For this review, use the dimensioned drawing (mm, ordinates from the lowest corner) and the shaded views. Coordinates: 2 decimals unless noted, no trailing zeros. Order: outer loops, then holes, each group sorted by start corner. A loop starts at its lowest first (then second) coordinate and runs counter-clockwise, first axis right, second up. Notation, with made-up numbers: M -33,1 L 18,1 A22 ccw 18,35 Z; hole C 76.25,69.5 d1. An arc over 180 degrees is marked long. Answer as CSV lines item,"result". Start each with the question number.
Q1. The part is to be moulded in two halves that separate along Y. For the marked faces 1, 2 and 3, say which applies: +Y half, -Y half, draft (parallel to the pull), parting line (faces both ways), or undercut.
Q2. For P1, Ø4, axis at x = 50.5, z = 34.5, coming from the -Y side; P2, Ø1.5, axis at x = 84, y = 220, coming from the +Z side; P3, Ø3, axis at x = 40, y = 187.5, coming from the +Z side, all flat-tipped, find the tip position at first contact; note any pin that passes through.
Q3. Wall thickness on L1, parallel to Y at x = 26, z = 150; L2, parallel to Y at x = 19.5, z = 120.5; L3, parallel to Z at x = 37, y = 148: over which ranges is each line inside the solid? List them lowest first. Write a range as [from, to].
Q4. Consider section A-A on z = 150. Write out the cut boundary in (x, y).
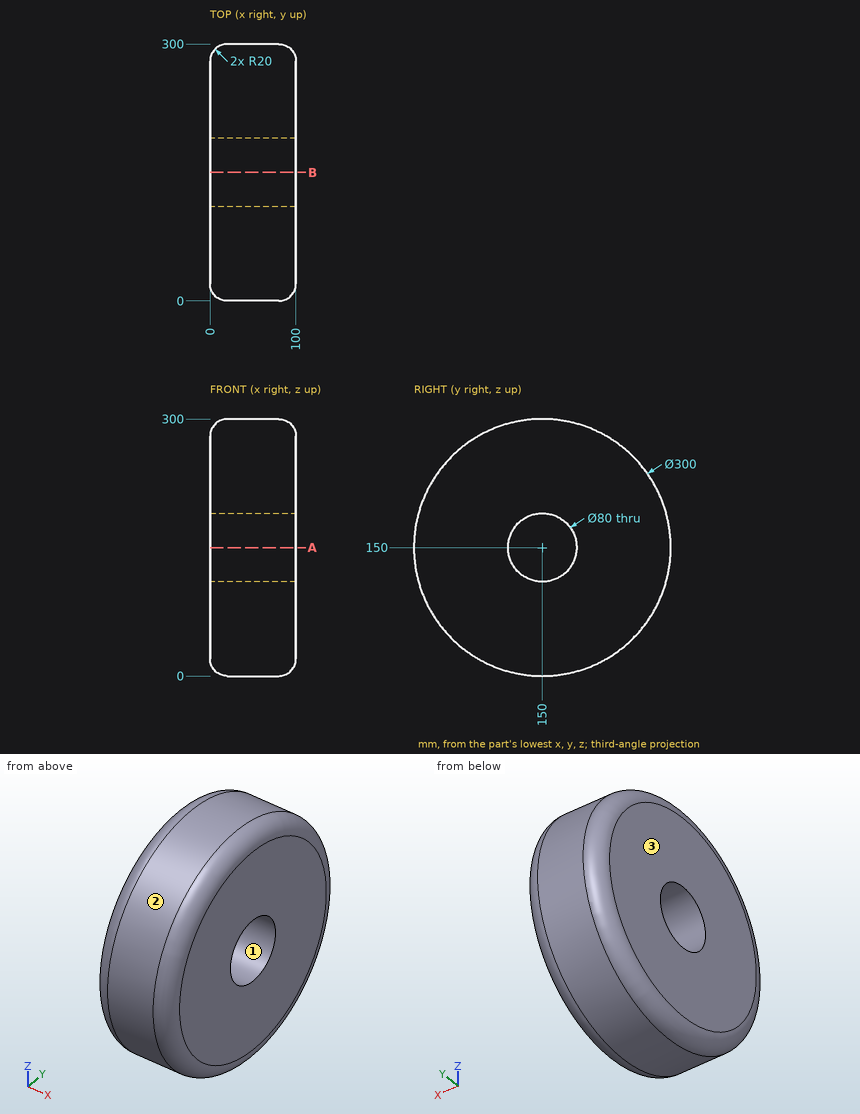
Evaluation:
1,face 1,"undercut"
1,face 2,"parting line"
1,face 3,"draft"
2,P1,"stops at y = 51.93"
2,P2,"stops at z = 282.64"
2,P3,"stops at z = 295.62"
3,L1,"y = [0, 110], [190, 300]"
3,L2,"y = [2.94, 122.99], [177.01, 297.06]"
3,L3,"z = [0.01, 110.05], [189.95, 299.99]"
4,outline,"M 0,20 A20 ccw 20,0 L 80,0 A20 ccw 100,20 L 100,110 L 0,110 Z; M 0,190 L 100,190 L 100,280 A20 ccw 80,300 L 20,300 A20 ccw 0,280 Z"
